from build123d import *

# Parameters (mm, degrees)
SKETCH_1_R      = 1
SKETCH_1_R_2    = 1.6
SKETCH_1_R_3    = 3.071217349
EXTRUDE_2_DEPTH = 3


with BuildPart() as part:
    # 草图1 → 凸台-拉伸2 (new body)
    with BuildSketch(Plane.XY):
        with BuildLine():
            Line((12, -8), (45.399810609, -8))
            ThreePointArc((45.399810609, -8), (59.25, -5), (45.399810609, -2))
            Line((45.399810609, -2), (12, -2))
            ThreePointArc((12, -2), (9, -5), (12, -8))
        make_face()
        with Locations((52, 0.5)):
            Circle(SKETCH_1_R, mode=Mode.SUBTRACT)
        with Locations((52, -10.5)):
            Circle(SKETCH_1_R, mode=Mode.SUBTRACT)
        with Locations((12, -5)):
            Circle(SKETCH_1_R_2, mode=Mode.SUBTRACT)
        with Locations((52, -5)):
            Circle(SKETCH_1_R_3, mode=Mode.SUBTRACT)
        with Locations((57.5, -5)):
            Circle(SKETCH_1_R, mode=Mode.SUBTRACT)
        with Locations((46.5, -5)):
            Circle(SKETCH_1_R, mode=Mode.SUBTRACT)
        with BuildLine():
            ThreePointArc((41.607192878, -6.5), (43.107192878, -5), (41.607192878, -3.5))
            Line((41.607192878, -3.5), (17.607192878, -3.5))
            ThreePointArc((17.607192878, -3.5), (16.107192878, -5), (17.607192878, -6.5))
            Line((17.607192878, -6.5), (41.607192878, -6.5))
        make_face(mode=Mode.SUBTRACT)
    extrude(amount=EXTRUDE_2_DEPTH)


solid = part.part
Here's how the part is built. I have some questions about the finished solid (model axes, mm). A direction names the side the tool comes from. Round coordinates to 2 decimals unless told otherwise and drop trailing zeros. Loops run counter-clockwise (first coordinate to the right, second up) from the corner with the lowest first, then second, coordinate; pieces in that order, holes last.
1. If I drill on line 1 along Y through (x, z) = (52, 2); line 2 along Y through (x, z) = (37.5, 2.85); line 3 along Y through (x, z) = (51.5, 1.5), over which ranges is the centre line in solid material (lowest first)?
Answer list:
line 1: y = -12.25 to -11.5, -9.5 to -8.07, -1.93 to -0.5, 1.5 to 2.25
line 2: y = -8 to -6.5, -3.5 to -2
line 3: y = -12.23 to -11.37, -9.63 to -8.03, -1.97 to -0.37, 1.37 to 2.23
2. Which directions (+Z, -Z, +X, -X, +Y, -Y) give clear straight access to the entire face, cutting with the end or side of a thin tool? Please do faces 1 (the face through (9, -5, 1)), 2 (the face through (29, -2, 1)), 3 (the face through (29, -6.5, 1)).
Answer list:
face 1: +Z, -Z, -X
face 2: +Z, -Z, -X, +Y
face 3: +Z, -Z
3. If we section it at B-B on z = 0.65: Write out the boundary of the cut face in (x, y), plus the area to 3 significant figures.
Answer list:
outline: (12, -8) - (45.4, -8) arc R7.25 ccw (long way) to (45.4, -2) - (12, -2) arc R3 ccw to start; hole circle Ø3.2 at (12, -5); hole (17.61, -6.5) - (41.61, -6.5) arc R1.5 ccw to (41.61, -3.5) - (17.61, -3.5) arc R1.5 ccw to start; hole circle Ø2 at (46.5, -5); hole circle Ø6.14 at (52, -5); hole circle Ø2 at (52, -10.5); hole circle Ø2 at (52, 0.5); hole circle Ø2 at (57.5, -5)
area: 248 mm2
4. If we section it at C-C on y = -5: Write out the boundary of the cut face in (x, z), plus the area to 3 significant figures.
Answer list:
outline: (9, 0) - (10.4, 0) - (10.4, 3) - (9, 3) - close; (13.6, 0) - (16.11, 0) - (16.11, 3) - (13.6, 3) - close; (43.11, 0) - (45.5, 0) - (45.5, 3) - (43.11, 3) - close; (47.5, 0) - (48.93, 0) - (48.93, 3) - (47.5, 3) - close; (55.07, 0) - (56.5, 0) - (56.5, 3) - (55.07, 3) - close; (58.5, 0) - (59.25, 0) - (59.25, 3) - (58.5, 3) - close
area: 29.7 mm2
5. We'd pull the mould along Y, two halves only. Please class faces 4 (the face through (59.245, -5.276, 1.479)), 5 (the face through (40, -3, 0)), 6 (the face through (51.263, 1.176, 1.479)), 7 (the face through (28, -8, 1)): +Y half, -Y half, draft (parallel to the pull), parting line (faces both ways), or undercut.
Answer list:
face 4: parting line
face 5: draft
face 6: undercut
face 7: -Y half
6. For P1, Ø0.9, axis at x = 30.5, z = 1.5, coming from the -Y side, with a flat end and sliding along its axis, tell me the tip position at first contact or that it passes through.
Answer list:
P1: stops at y = -8
7. If we section it at D-D on y = 1: Write out the boundary of the cut face in (x, z), plus the area to 3 significant figures.
Answer list:
outline: (47.93, 0) - (51.13, 0) - (51.13, 3) - (47.93, 3) - close; (52.87, 0) - (56.07, 0) - (56.07, 3) - (52.87, 3) - close
area: 19.2 mm2
8. If we section it at A-A on x = 52: Write out the boundary of the cut face in (y, z), plus the area to 3 significant figures.
Answer list:
outline: (-12.25, 0) - (-11.5, 0) - (-11.5, 3) - (-12.25, 3) - close; (-9.5, 0) - (-8.07, 0) - (-8.07, 3) - (-9.5, 3) - close; (-1.93, 0) - (-0.5, 0) - (-0.5, 3) - (-1.93, 3) - close; (1.5, 0) - (2.25, 0) - (2.25, 3) - (1.5, 3) - close
area: 13.1 mm2
